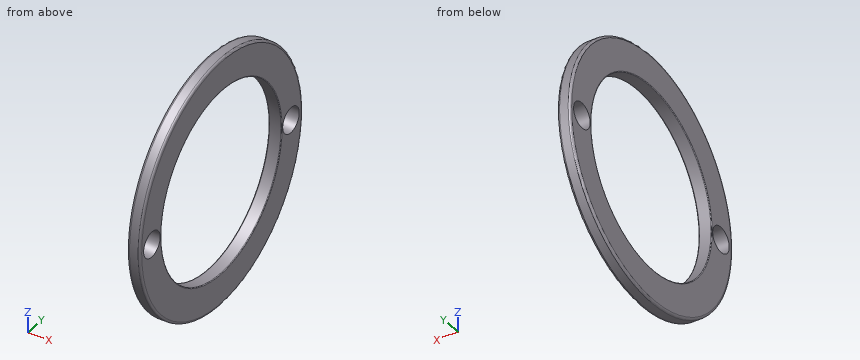
```python
from build123d import *

# Parameters (mm, degrees)
CROQUIS2_R     = 3.572
EXTRUIR1_DEPTH = 12.358
CROQUIS3_R     = 3.572
EXTRUIR2_DEPTH = 12.358


with BuildPart() as part:
    # Croquis1 → Revolución1 (revolve)
    with BuildSketch(Plane.XY):
        with BuildLine():
            Line((5.214, 34.4), (5.214, 26.2))
            ThreePointArc((5.214, 26.2), (5.272578644, 26.058578644), (5.414, 26))
            Line((5.414, 26), (8.586, 26))
            ThreePointArc((8.586, 26), (8.727421356, 26.058578644), (8.786, 26.2))
            Line((8.786, 26.2), (8.786, 34.4))
            ThreePointArc((8.786, 34.4), (8.610264069, 34.824264069), (8.186, 35))
            Line((8.186, 35), (5.814, 35))
            ThreePointArc((5.814, 35), (5.389735931, 34.824264069), (5.214, 34.4))
        make_face()
    revolve(axis=Axis((50, 0, 0), (-1, 0, 0)))

    # Croquis2 → Extruir1 (cut)
    with BuildSketch(Plane(origin=(0, 0, 0), x_dir=(0, 0, -1), z_dir=(1, 0, 0))):
        with Locations((0, 30)):
            Circle(CROQUIS2_R)
    extrude(amount=EXTRUIR1_DEPTH, mode=Mode.SUBTRACT)

    # Croquis3 → Extruir2 (cut)
    with BuildSketch(Plane(origin=(0, 0, 0), x_dir=(0, 0, -1), z_dir=(1, 0, 0))):
        with Locations((0, -30)):
            Circle(CROQUIS3_R)
    extrude(amount=EXTRUIR2_DEPTH, mode=Mode.SUBTRACT)


solid = part.part
```
Can you work these out from the model? Positions are in its coordinate system, mm. Coordinates: 2 decimals unless noted, no trailing zeros. Loops run counter-clockwise (first coordinate to the right, second up) from the corner with the lowest first, then second, coordinate; pieces in that order, holes last. Notation, with made-up numbers: (83.5, -33.75) - (90.5, -33.75) arc R12 ccw to (90.5, -28.75) - close; hole circle Ø11 at (11, 2.25). An arc over 180 degrees is marked (long way). Answer as CSV lines item,"result". Start each with the question number.
1) I need wall thicknesses on line 1 (Y direction, x = 6.7, z = 0); line 2 (Z direction, x = 7.6, y = 0); line 3 (Y direction, x = 7.1, z = -1). Which ranges of each line are inside material? Lowest first, please. Write a range as from..to.
2) Suppose I cut it at C-C (x = 6.6). Please give me the cut outline in (y, z), plus the area to 3 significant figures.
3) Suppose I cut it at A-A (y = 0). Please give me the cut outline in (x, z), plus the area to 3 significant figures.
4) For pin 1 (1.5 mm diameter, centred on x = 6, z = 20.5, fed in from +Y); pin 2 (1 mm diameter, centred on x = 6.5, y = 4.5, fed in from +Z); pin 3 (1 mm diameter, centred on x = 7.5, z = -25, fed in from +Y) (3 decimals), each with a flat end and sliding along its axis, tell me the tip position at first contact or that it passes through.
5) Suppose I cut it at B-B (z = 0). Please give me the cut outline in (x, y).
Check result:
1,line 1,"y = -35..-33.57, -26.43..-26, 26..26.43, 33.57..35"
1,line 2,"z = -35..-26, 26..35"
1,line 3,"y = -34.99..-33.43, -26.57..-25.98, 25.98..26.57, 33.43..34.99"
2,outline,"circle Ø70 at (0, 0); hole circle Ø7.14 at (-30, 0); hole circle Ø52 at (0, 0); hole circle Ø7.14 at (30, 0)"
2,area,"1,640 mm²"
3,outline,"(5.21, -34.4) arc R0.6 ccw to (5.81, -35) - (8.19, -35) arc R0.6 ccw to (8.79, -34.4) - (8.79, -26.2) arc R0.2 ccw to (8.59, -26) - (5.41, -26) arc R0.2 ccw to (5.21, -26.2) - close; (5.21, 26.2) arc R0.2 ccw to (5.41, 26) - (8.59, 26) arc R0.2 ccw to (8.79, 26.2) - (8.79, 34.4) arc R0.6 ccw to (8.19, 35) - (5.81, 35) arc R0.6 ccw to (5.21, 34.4) - close"
3,area,"64.0 mm²"
4,pin 1,"stops at y = 28.9"
4,pin 2,"stops at z = 34.77"
4,pin 3,"stops at y = 24.995"
5,outline,"(5.21, -34.4) arc R0.6 ccw to (5.81, -35) - (8.19, -35) arc R0.6 ccw to (8.79, -34.4) - (8.79, -33.57) - (5.21, -33.57) - close; (5.21, -26.43) - (8.79, -26.43) - (8.79, -26.2) arc R0.2 ccw to (8.59, -26) - (5.41, -26) arc R0.2 ccw to (5.21, -26.2) - close; (5.21, 26.2) arc R0.2 ccw to (5.41, 26) - (8.59, 26) arc R0.2 ccw to (8.79, 26.2) - (8.79, 26.43) - (5.21, 26.43) - close; (5.21, 33.57) - (8.79, 33.57) - (8.79, 34.4) arc R0.6 ccw to (8.19, 35) - (5.81, 35) arc R0.6 ccw to (5.21, 34.4) - close"
